from build123d import *

# Parameters (mm, degrees)
SKETCH_1_W          = 215
SKETCH_1_H          = 115
EXTRUDE_1_DEPTH     = 50
SKETCH_2_W          = 25
SKETCH_2_H          = 111
CUT_EXTRUDE_1_DEPTH = 45
CUT_EXTRUDE_3_DEPTH = 15


with BuildPart() as part:
    # Эскиз1 → Бобышка-Вытянуть1 (new body)
    with BuildSketch(Plane(origin=(0, 0, 0), x_dir=(1, 0, 0), z_dir=(0, 1, 0))):
        with Locations((107.5, 57.5)):
            Rectangle(SKETCH_1_W, SKETCH_1_H)
    extrude(amount=EXTRUDE_1_DEPTH)

    # Эскиз2 → Вырез-Вытянуть1 (cut)
    with BuildSketch(Plane(origin=(0, 50, 0), x_dir=(1, 0, 0), z_dir=(0, 1, 0))):
        with Locations((202.5, 57.5)):
            Rectangle(SKETCH_2_W, SKETCH_2_H)
    extrude(amount=-CUT_EXTRUDE_1_DEPTH, mode=Mode.SUBTRACT)

    # Эскиз3 → Вырез-Вытянуть3 (cut)
    with BuildSketch(Plane(origin=(0, 50, 0), x_dir=(1, 0, 0), z_dir=(0, 1, 0))):
        with BuildLine():
            ThreePointArc((36.6, 23.343469749), (40, 23), (43.4, 23.343469749))
            ThreePointArc((43.4, 23.343469749), (44.959591794, 25.703061543), (42.6, 27.262653338))
            ThreePointArc((42.6, 27.262653338), (40, 27), (37.4, 27.262653338))
            ThreePointArc((37.4, 27.262653338), (35.040408206, 25.703061543), (36.6, 23.343469749))
        make_face()
        with BuildLine():
            ThreePointArc((23.875021664, 34.616221247), (25.277568136, 31.5), (27.275021664, 28.727248502))
            ThreePointArc((27.275021664, 28.727248502), (30.098283997, 28.556398285), (30.269134213, 31.379660619))
            ThreePointArc((30.269134213, 31.379660619), (28.741669751, 33.5), (27.669134213, 35.882992719))
            ThreePointArc((27.669134213, 35.882992719), (25.138692203, 37.146663258), (23.875021664, 34.616221247))
        make_face()
        with BuildLine():
            ThreePointArc((27.275021664, 51.272751498), (25.277568136, 48.5), (23.875021664, 45.383778753))
            ThreePointArc((23.875021664, 45.383778753), (25.138692203, 42.853336742), (27.669134213, 44.117007281))
            ThreePointArc((27.669134213, 44.117007281), (28.741669751, 46.5), (30.269134213, 48.620339381))
            ThreePointArc((30.269134213, 48.620339381), (30.098283997, 51.443601715), (27.275021664, 51.272751498))
        make_face()
        with BuildLine():
            ThreePointArc((43.4, 56.656530251), (40, 57), (36.6, 56.656530251))
            ThreePointArc((36.6, 56.656530251), (35.040408206, 54.296938457), (37.4, 52.737346662))
            ThreePointArc((37.4, 52.737346662), (40, 53), (42.6, 52.737346662))
            ThreePointArc((42.6, 52.737346662), (44.959591794, 54.296938457), (43.4, 56.656530251))
        make_face()
        with BuildLine():
            ThreePointArc((56.124978336, 45.383778753), (54.722431864, 48.5), (52.724978336, 51.272751498))
            ThreePointArc((52.724978336, 51.272751498), (49.901716003, 51.443601715), (49.730865787, 48.620339381))
            ThreePointArc((49.730865787, 48.620339381), (51.258330249, 46.5), (52.330865787, 44.117007281))
            ThreePointArc((52.330865787, 44.117007281), (54.861307797, 42.853336742), (56.124978336, 45.383778753))
        make_face()
        with BuildLine():
            ThreePointArc((52.724978336, 28.727248502), (54.722431864, 31.5), (56.124978336, 34.616221247))
            ThreePointArc((56.124978336, 34.616221247), (54.861307797, 37.146663258), (52.330865787, 35.882992719))
            ThreePointArc((52.330865787, 35.882992719), (51.258330249, 33.5), (49.730865787, 31.379660619))
            ThreePointArc((49.730865787, 31.379660619), (49.901716003, 28.556398285), (52.724978336, 28.727248502))
        make_face()
        with BuildLine():
            ThreePointArc((33.466666667, 16.387173918), (40, 15.5), (46.533333333, 16.387173918))
            ThreePointArc((46.533333333, 16.387173918), (47.927577639, 18.848084891), (45.466666667, 20.242329197))
            ThreePointArc((45.466666667, 20.242329197), (40, 19.5), (34.533333333, 20.242329197))
            ThreePointArc((34.533333333, 20.242329197), (32.072422361, 18.848084891), (33.466666667, 16.387173918))
        make_face()
        with BuildLine():
            ThreePointArc((16.284026092, 33.851619597), (18.782377607, 27.75), (22.817359425, 22.535554321))
            ThreePointArc((22.817359425, 22.535554321), (25.645692997, 22.558558819), (25.622688498, 25.386892391))
            ThreePointArc((25.622688498, 25.386892391), (22.246479222, 29.75), (20.156021832, 34.855436806))
            ThreePointArc((20.156021832, 34.855436806), (17.718115357, 36.289526072), (16.284026092, 33.851619597))
        make_face()
        with BuildLine():
            ThreePointArc((22.817359425, 57.464445679), (18.782377607, 52.25), (16.284026092, 46.148380403))
            ThreePointArc((16.284026092, 46.148380403), (17.718115357, 43.710473928), (20.156021832, 45.144563194))
            ThreePointArc((20.156021832, 45.144563194), (22.246479222, 50.25), (25.622688498, 54.613107609))
            ThreePointArc((25.622688498, 54.613107609), (25.645692997, 57.441441181), (22.817359425, 57.464445679))
        make_face()
        with BuildLine():
            ThreePointArc((46.533333333, 63.612826082), (40, 64.5), (33.466666667, 63.612826082))
            ThreePointArc((33.466666667, 63.612826082), (32.072422361, 61.151915109), (34.533333333, 59.757670803))
            ThreePointArc((34.533333333, 59.757670803), (40, 60.5), (45.466666667, 59.757670803))
            ThreePointArc((45.466666667, 59.757670803), (47.927577639, 61.151915109), (46.533333333, 63.612826082))
        make_face()
        with BuildLine():
            ThreePointArc((63.715973908, 46.148380403), (61.217622393, 52.25), (57.182640575, 57.464445679))
            ThreePointArc((57.182640575, 57.464445679), (54.354307003, 57.441441181), (54.377311502, 54.613107609))
            ThreePointArc((54.377311502, 54.613107609), (57.753520778, 50.25), (59.843978168, 45.144563194))
            ThreePointArc((59.843978168, 45.144563194), (62.281884643, 43.710473928), (63.715973908, 46.148380403))
        make_face()
        with BuildLine():
            ThreePointArc((57.182640575, 22.535554321), (61.217622393, 27.75), (63.715973908, 33.851619597))
            ThreePointArc((63.715973908, 33.851619597), (62.281884643, 36.289526072), (59.843978168, 34.855436806))
            ThreePointArc((59.843978168, 34.855436806), (57.753520778, 29.75), (54.377311502, 25.386892391))
            ThreePointArc((54.377311502, 25.386892391), (54.354307003, 22.558558819), (57.182640575, 22.535554321))
        make_face()
    extrude(amount=-CUT_EXTRUDE_3_DEPTH, mode=Mode.SUBTRACT)


solid = part.part
Build history of the part. All positions in model axes, mm. A direction names the side the tool comes from. Round coordinates to 2 decimals unless told otherwise and drop trailing zeros. Loops run counter-clockwise (first coordinate to the right, second up) from the corner with the lowest first, then second, coordinate; pieces in that order, holes last. Notation, with made-up numbers: (62.25, 36) -> (81.25, 36) arc R20 cw to (81.25, 73) -> close; hole circle Ø5 at (39, 71.5). An arc over 180 degrees is marked (long way). Use CSV: the item, a comma, the result in double quotes. Start each with the question number.
Q1. Drill centre lines: L1, parallel to X at y = 39, z = -57.5; L2, parallel to Z at x = 192, y = 11.5; L3, parallel to Z at x = 21, y = 36.5. Where is each one in solid material? Low to high.
Q2. Flat gauge pins, fed straight in: pin 1 Ø7.5 at (x, y) = (208, 23) entering from +Z; pin 2 Ø10 at (y, z) = (41.5, -46) entering from +X; pin 3 Ø1.3 at (x, z) = (37.5, -54.5) entering from +Y. Where does each tip first touch, or does it go through?
Q3. Saw through at A-A on y = 30. Give the cut face in (x, z), and give its area (4 significant figures).
Q4. Mould opens along Z. For faces 4 (the face through (22.208, 42.605, -50.183)), 5 (the face through (106, 25, -115)), 6 (the face through (106, 0, -58)) say: +Z half, -Z half, draft (parallel to the pull), parting line (faces both ways), or undercut.
Q5. Which spindle directions (+Z, -Z, +X, -X, +Y, -Y) get a long thin tool onto all of the face, cutting with end or side? Do faces 1 (the face through (0, 25, -57)), 2 (the face through (40, 43, -23)), 3 (the face through (202, 5, -58)). Say none if no direction does.
Solutions:
1,L1,"x = 0 to 22.85, 25.59 to 54.41, 57.15 to 190"
1,L2,"z = -115 to -113, -2 to 0"
1,L3,"z = -115 to -55.47, -47.7 to -32.3, -24.53 to 0"
2,pin 1,"stops at z = 0"
2,pin 2,"stops at x = 190"
2,pin 3,"stops at y = 35"
3,outline,"(0, -115) -> (215, -115) -> (215, -113) -> (190, -113) -> (190, -2) -> (215, -2) -> (215, 0) -> (0, 0) -> close"
3,area,"21,950 mm^2"
4,face 4,"undercut"
4,face 5,"-Z half"
4,face 6,"draft"
5,face 1,"+Z, -Z, -X, +Y, -Y"
5,face 2,"+Y"
5,face 3,"+X, +Y"
